Can you work these out from the drawing? Everything is in mm from the part's minimum corner. A direction names the side the tool comes from. Give positions to 0.01 mm unless a question says otherwise; leave off trailing zeros. Order: outer loops, then holes, each group sorted by start corner. A loop starts at its lowest first (then second) coordinate and runs counter-clockwise, first axis right, second up. Notation, with made-up numbers: (68, 18.5) - (74, 18.5) arc R28 cw to (74, 56.5) - close; hole circle Ø4 at (1, -18.75). An arc over 180 degrees is marked (long way). Write each question's results on one line, items separated by ' | '. Start each with the question number.
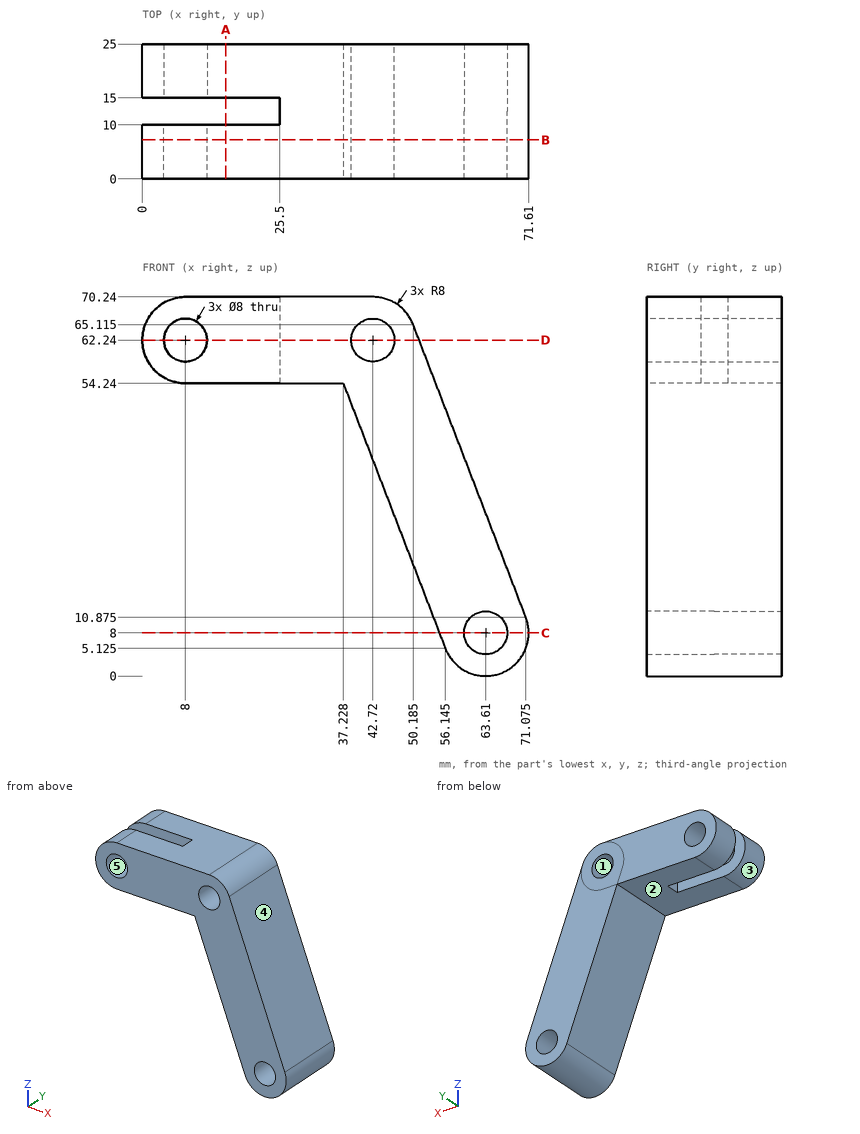
Q1. If we section it at B-B (y = 7.25): Please give me the cut outline in (x, z) (1 decimal).
Q2. If we section it at D-D (z = 62.24): Please give me the cut outline in (x, y), plus the area to 3 significant figures.
Q3. Will these pins go through, and if not, where does the flat tip stop? P1, Ø2.5, axis at y = 11.5, z = 61, coming from the -X side; P2, Ø13, axis at x = 14.5, z = 63, coming from the -Y side; P3, Ø5, axis at y = 15.5, z = 58, coming from the +X side; P4, Ø7.5, axis at x = 18, y = 9.5, coming from the -Z side.
Q4. If we section it at A-A (x = 15.5): Please give me the cut outline in (y, z), plus the area to 3 significant figures.
Q5. Which directions (+Z, -Z, +X, -X, +Y, -Y) give clear straight access to the entire face, cutting with the end or side of a thin tool? Please do the marked faces 1 and 2.
Q6. If we section it at C-C (z = 8): Please give me the cut outline in (x, y).
Q7. Thinking about a two-plate mould opening in Z: for the marked faces 3, 4 and 5, which applies, released by +Z, released by -Z, zero draft, split by the parting line, or undercut?
Q8. If I drill on probe 1 along X at (y, z) = (7.25, 62.24); probe 2 along X at (y, z) = (23.75, 59) (1 decimal); probe 3 along Z at (x, y) = (8, 20.75), over which ranges is the centre line in solid material (lowest first)? Write a range as from..to.
Findings below:
1) outline: (8, 54.2) - (37.2, 54.2) - (56.1, 5.1) arc R8 ccw to (71.1, 10.9) - (50.2, 65.1) arc R8 ccw to (42.7, 70.2) - (8, 70.2) arc R8 ccw to start; hole circle Ø8 at (8, 62.2); hole circle Ø8 at (42.7, 62.2); hole circle Ø8 at (63.6, 8)
2) outline: (0, 0) - (4, 0) - (4, 10) - (0, 10) - close; (0, 15) - (4, 15) - (4, 25) - (0, 25) - close; (12, 0) - (38.72, 0) - (38.72, 25) - (12, 25) - (12, 15) - (25.5, 15) - (25.5, 10) - (12, 10) - close; (46.72, 0) - (51.29, 0) - (51.29, 25) - (46.72, 25) - close | area: 795 mm2
3) P1: stops at x = 25.5 | P2: stops at y = 0 | P3: stops at x = 53.89 | P4: stops at z = 54.24
4) outline: (0, 54.24) - (10, 54.24) - (10, 70.24) - (0, 70.24) - close; (15, 54.24) - (25, 54.24) - (25, 70.24) - (15, 70.24) - close | area: 320 mm2
5) face 1: +Y, -Y | face 2: -Z, -X, +Y, -Y
6) outline: (55.04, 0) - (59.61, 0) - (59.61, 25) - (55.04, 25) - close; (67.61, 0) - (71.61, 0) - (71.61, 25) - (67.61, 25) - close
7) face 3: split by the parting line | face 4: released by +Z | face 5: undercut
8) probe 1: x = 0..4, 12..38.72, 46.72..51.29 | probe 2: x = 0.7..5.7, 10.3..40.4, 45.1..52.5 | probe 3: z = 54.24..58.24, 66.24..70.24
